Autodesk Inventor part; units mm, degrees
ref_plane "YZ Plane" through (0, 0, 0) normal (1, 0, 0) x (0, 1, 0)
ref_plane "XZ Plane" through (0, 0, 0) normal (0, 1, 0) x (-1, 0, 0)
ref_plane "XY Plane" through (0, 0, 0) normal (0, 0, 1) x (1, 0, 0)
sketch "Sketch1" plane through (0, 0, 0) normal (0, 0, 1) x (1, 0, 0)
  point P0 (0, 0)
sketch "Sketch2" plane through (0, 0, 0) normal (0, 1, 0) x (-1, 0, 0)
  line L0 (0, 0) -> (0, -9)
  line L1 (0, -9) -> (-2.5, -9)
  line L2 (-2.5, -9) -> (-2.5, -2.5)
  line L3 (-2.5, -2.5) -> (-9, -2.5)
  line L4 (-9, -2.5) -> (-9, 0)
  line L5 (-9, 0) -> (0, 0)
  dimension "d0" = 9
  dimension "d1" = 2.5
  dimension "d2" = 9
  dimension "d3" = 2.5
extrude "Extrusion1" add sketch "Sketch2" against normal blind 23
sketch "Sketch3" plane through (0, 0, 0) normal (0, 0, 1) x (1, 0, 0)
  circle A0 centre (5.5, -11.5) radius 1.5
  line L0 (0, 0) -> (9, 0)
  line L1 (0, 0) -> (0, -23)
  dimension "d6" = 3
  dimension "d7" = 11.5
  dimension "d8" = 5.5
extrude "Extrusion2" cut sketch "Sketch3" against normal blind 23
sketch "Sketch4" plane through (0, 0, -9) normal (-1, 0, 0) x (0, 0, 1)
  circle A0 centre (3.5, -5.5) radius 1.5
  circle A1 centre (3.5, -17.5) radius 1.5
  line L0 (0, 0) -> (9, 0)
  line L1 (9, -23) -> (0, -23)
  line L2 (9, 0) -> (9, -23)
  dimension "d11" = 3
  dimension "d12" = 3
  dimension "d13" = 5.5
  dimension "d14" = 5.5
  dimension "d15" = 12
  dimension "d16" = 5.5
extrude "Extrusion3" cut sketch "Sketch4" against normal blind 23
fillet "Fillet1" radius 1 4 edges at (1.25, 0, -9) (9, 0, -1.25) (9, -23, -1.25) (1.25, -23, -9)
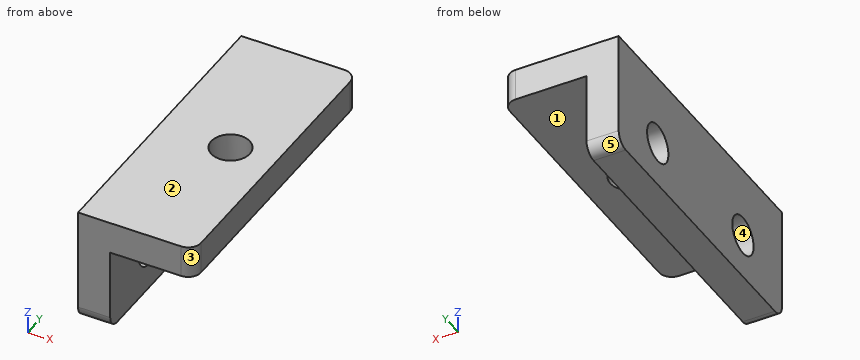
Here's how the part is built. I have some questions about the finished solid (model axes, mm). Face numbers are marked on the shaded views. A direction names the side the tool comes from. Give positions to 0.01 mm unless a question says otherwise; leave off trailing zeros. Loops run counter-clockwise (first coordinate to the right, second up) from the corner with the lowest first, then second, coordinate; pieces in that order, holes last. Notation, with made-up numbers: M -8.5,9 L 21.5,9 A30 ccw 21.5,31 Z; hole C 46.25,50 d5. An arc over 180 degrees is marked long. Return JSON: item names as keys, results as strings.
Item 1: I'm going to push flat-ended pins straight in: pin 1 Ø1.8 at (x, y) = (5.5, -11.5) entering from -Z; pin 2 Ø3 at (y, z) = (-12, -6.5) entering from +X; pin 3 Ø2 at (x, y) = (7, -13) entering from -Z. Where does each tip first touch, or does it pass through?
A:
{"pin 1": "passes through", "pin 2": "stops at x = 2.5", "pin 3": "stops at z = -2.5"}
Item 2: Imagine slicing it at C-C on z = -1. List the corners of the cut face in (x, y) for me, then the cut area to 3 significant figures.
A:
{"outline": "M 0,-23 L 8,-23 A1 ccw 9,-22 L 9,-1 A1 ccw 8,0 L 0,0 Z; hole C 5.5,-11.5 d3", "area": "200 mm^2"}
Item 3: Please list where these lines run through material, in increasing order: line 1 (Y direction, x = 0.8, z = -5.5); line 2 (Y direction, x = 0.75, z = -4.5); line 3 (X direction, y = -20.5, z = -6.25).
A:
{"line 1": "y = -23 to -19, -16 to -7, -4 to 0", "line 2": "y = -23 to -18.62, -16.38 to -6.62, -4.38 to 0", "line 3": "x = 0 to 2.5"}
Item 4: Thinking about a two-plate mould opening in Y: for the marked faces 3, 4 and 5, which applies, released by +Y, released by -Y, zero draft, split by the parting line, or undercut?
A:
{"face 3": "released by -Y", "face 4": "undercut", "face 5": "released by +Y"}
Item 5: Imagine slicing it at A-A on z = -5.5. List the corners of the cut face in (x, y) for me.
A:
{"outline": "M 0,-23 L 2.5,-23 L 2.5,-19 L 0,-19 Z; M 0,-16 L 2.5,-16 L 2.5,-7 L 0,-7 Z; M 0,-4 L 2.5,-4 L 2.5,0 L 0,0 Z"}
Item 6: On a 3-axis mill with a long thin cutter (end or side, diameter ignored), from which of +Z, -Z, +X, -X, +Y, -Y can I reach the whole of each face in a straight line? I mean the marked faces 1 and 2. Say none if no direction works.
A:
{"face 1": "-Z, +X, +Y, -Y", "face 2": "+Z, +X, -X, +Y, -Y"}
Item 7: Imagine slicing it at D-D on y = -14. List the corners of the cut face in (x, z) for me, then the cut area to 4 significant figures.
A:
{"outline": "M 0,-9 L 2.5,-9 L 2.5,-2.5 L 9,-2.5 L 9,0 L 0,0 Z", "area": "38.75 mm^2"}
Item 8: Imagine slicing it at B-B on y = -11.5. List the corners of the cut face in (x, z) for me.
A:
{"outline": "M 0,-9 L 2.5,-9 L 2.5,-2.5 L 4,-2.5 L 4,0 L 0,0 Z; M 7,-2.5 L 9,-2.5 L 9,0 L 7,0 Z"}
